```python
from build123d import *

# Parameters (mm, degrees)
F0_R     = 6
F1_DEPTH = 3
F1_TAPER = -45
F2_DEPTH = 40
F4_DEPTH = 5


with BuildPart() as f1:
    # F0 (on Top) → F1 (new body)
    with BuildSketch(Plane.XY):
        Circle(F0_R)
    extrude(amount=F1_DEPTH, taper=F1_TAPER)

    # F0 (on Top) → F2 (join)
    with BuildSketch(Plane.XY):
        Circle(F0_R)
    extrude(amount=-F2_DEPTH)

    # F3 (on face) → F4 (cut)
    with BuildSketch(Plane.XY.offset(3)):
        Polygon((2.6050036522, -4.5119986795), (5.2100073044, 0), (2.6050036522, 4.5119986795), (-2.6050036522, 4.5119986795), (-5.2100073044, 0), (-2.6050036522, -4.5119986795), align=None)
    extrude(amount=-F4_DEPTH, mode=Mode.SUBTRACT)


solid = f1.part
```
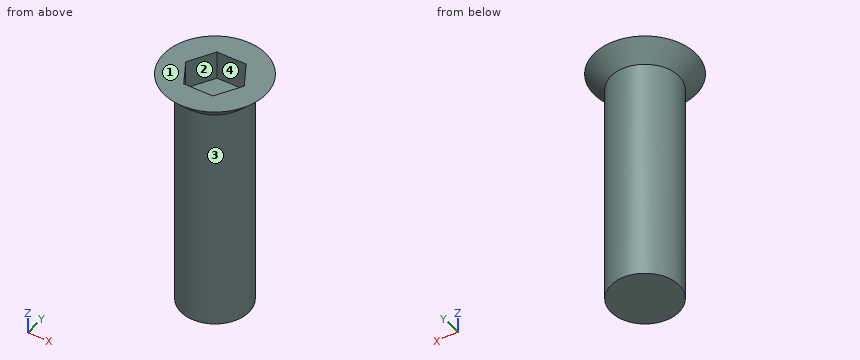
Work out the finished part from the listing and answer in its coordinate system (mm). Face numbers are marked on the shaded views. Give positions to 0.01 mm unless a question says otherwise; leave off trailing zeros. Write each loop counter-clockwise with the first axis right and the second up, starting at its lowest first coordinate (ties: lowest second). Pieces come first, ordered by that corner, then holes. Notation, with made-up numbers: (-21.5, 3) - (18.5, 3) arc R27 ccw to (18.5, 25) - close; hole circle Ø6 at (-25, 30). An arc over 180 degrees is marked (long way). Use one line per item in the form item = value.
1. Consider L1, parallel to Z at x = 1.25, y = 2; L2, parallel to Y at x = 0, z = -17; L3, parallel to X at y = -5.25, z = -24.5. Determine where each line is inside the solid, lowest interval first.
Filled in:
L1 = -40 to -2
L2 = -6 to 6
L3 = -2.9 to 2.9
2. Each of these flat-tipped pins is pushed along its axis until it touches: pin 1 Ø5.5 at (x, z) = (-1, -0.5) entering from -Y; pin 2 Ø4 at (x, z) = (-3.5, -4.5) entering from +Y; pin 3 Ø2.5 at (x, y) = (0.5, 1.5) entering from +Z. Where does it stop, or does it pass through?
Filled in:
pin_1 = -8.2
pin_2 = 5.81
pin_3 = -2
3. Determine the mould class of the marked faces 1, 2, 3 and 4 for opening direction Y: released by +Y, released by -Y, zero draft, split by the parting line, or undercut.
Filled in:
face_1 = zero draft
face_2 = undercut
face_3 = split by the parting line
face_4 = undercut
4. A cutting plane is placed at B-B (z = -21.5). Write down the section's boundary in (x, y).
Filled in:
outline = circle Ø12 at (0, 0)
5. A cutting plane is placed at A-A (x = 0). Write down the section's boundary in (y, z).
Filled in:
outline = (-9, 3) - (-6, 0) - (-6, -40) - (6, -40) - (6, 0) - (9, 3) - (4.51, 3) - (4.51, -2) - (-4.51, -2) - (-4.51, 3) - close
